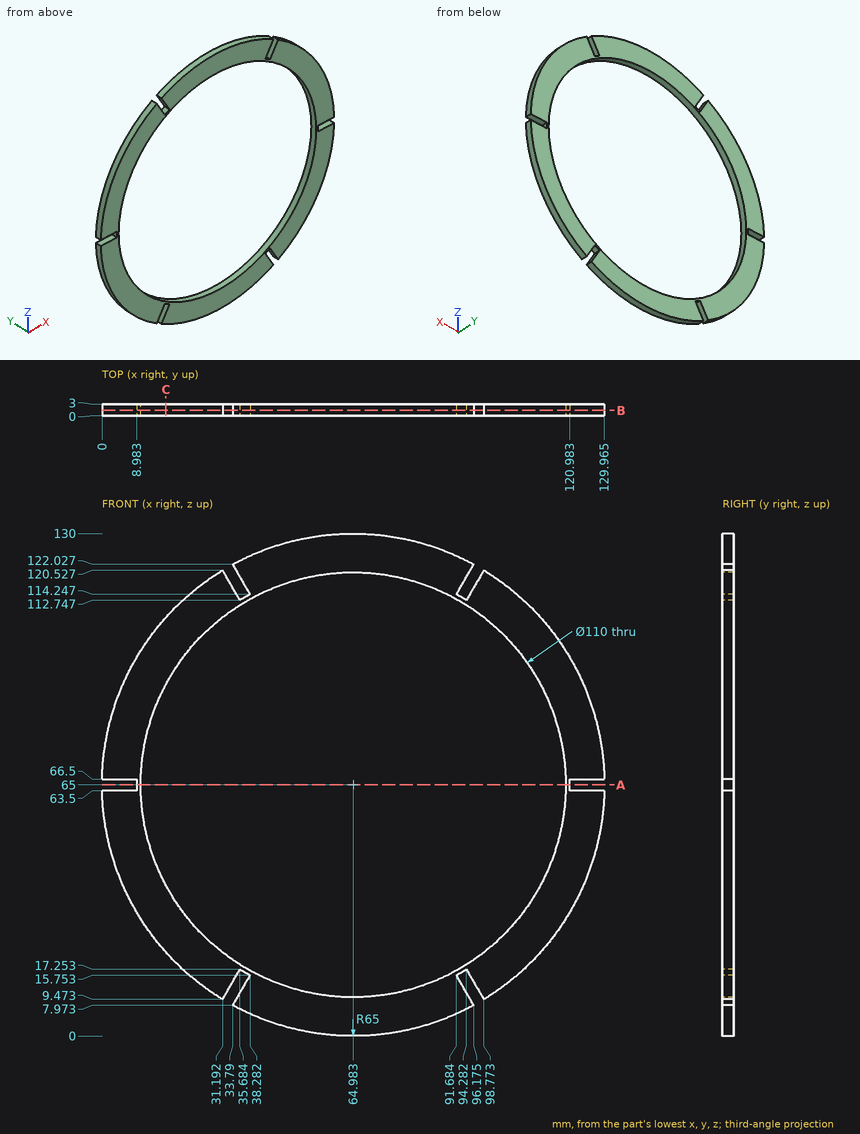
The figure shows three views and two pictorial views of one solid part (mm, origin at its lowest corner). Answer the questions. Coordinates: 2 decimals unless noted, no trailing zeros. Loops run counter-clockwise (first coordinate to the right, second up) from the corner with the lowest first, then second, coordinate; pieces in that order, holes last.
1) Find the intervals of material crossed by L1, parallel to X at y = 1.3, z = 65.5 (1 decimal); L2, parallel to Z at x = 44, y = 2.75; L3, parallel to Z at x = 83.5, y = 0.55, in increasing order.
2) Find section B-B on y = 1.35. Write down the section's boundary in (x, z) (1 decimal).
3) Find section A-A on z = 65. Write down the section's boundary in (x, y).
4) Flat-ended cylindrical pins translate along their axes: pin 1 Ø1.5 at (y, z) = (2, 65) entering from +X; pin 2 Ø1.5 at (x, y) = (123.5, 1.5) entering from +Z. Find the tip coordinate at first contact, or state that the pin passes through.
5) Find section C-C on x = 16.5. Write down the section's boundary in (y, z) (1 decimal), then the cut area to 3 significant figures.
Values:
1. L1: x = 9 to 10, 120 to 121
1. L2: z = 3.48 to 14.16, 115.84 to 126.52
1. L3: z = 2.69 to 13.21, 116.79 to 127.31
2. outline: (0, 63.5) arc R65 ccw to (31.2, 9.5) - (35.7, 17.3) - (38.3, 15.8) - (33.8, 8) arc R65 ccw to (96.2, 8) - (91.7, 15.8) - (94.3, 17.3) - (98.8, 9.5) arc R65 ccw to (130, 63.5) - (121, 63.5) - (121, 66.5) - (130, 66.5) arc R65 ccw to (98.8, 120.5) - (94.3, 112.7) - (91.7, 114.2) - (96.2, 122) arc R65 ccw to (33.8, 122) - (38.3, 114.2) - (35.7, 112.7) - (31.2, 120.5) arc R65 ccw to (0, 66.5) - (9, 66.5) - (9, 63.5) - close; hole circle Ø110 at (65, 65)
3. outline: (8.98, 0) - (9.98, 0) - (9.98, 3) - (8.98, 3) - close; (119.98, 0) - (120.98, 0) - (120.98, 3) - (119.98, 3) - close
4. pin 1: stops at x = 120.98
4. pin 2: stops at z = 94.8
5. outline: (0, 21.7) - (3, 21.7) - (3, 39) - (0, 39) - close; (0, 91) - (3, 91) - (3, 108.3) - (0, 108.3) - close
5. area: 104 mm2
